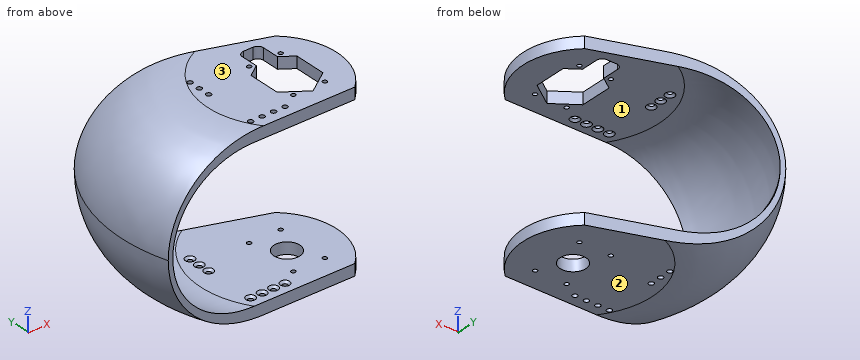
from build123d import *

# Parameters (mm, degrees)
SKETCH1_R                                          = 14.287500000000003
SKETCH1_R_2                                        = 2.3812500000000005
SKETCH1_R_3                                        = 2.3812500000000023
BOSS_EXTRUDE1_DEPTH                                = 190.5
CUT_EXTRUDE1_DEPTH                                 = 314.11990818452256
BOSS_EXTRUDE2_DEPTH                                = 165.1
CUT_EXTRUDE3_REACH                                 = 289.993
FILLET2_R                                          = 82.296
FILLET3_R                                          = 95.25
CSK_FOR_10_FLAT_HEAD_MACHINE_SCREW_100_D           = 5.6134
CSK_FOR_10_FLAT_HEAD_MACHINE_SCREW_100_DEPTH       = 21.30479447
CSK_FOR_10_FLAT_HEAD_MACHINE_SCREW_100_CSINK_D     = 10.16
CSK_FOR_10_FLAT_HEAD_MACHINE_SCREW_100_CSINK_ANGLE = 90


with BuildPart() as part:
    # Sketch1 → Boss-Extrude1 (new body)
    with BuildSketch(Plane.XY):
        with BuildLine():
            Line((31.75000000000027, -53.33999999999999), (-174.9283819167147, -53.33999999999997))
            ThreePointArc((-174.9283819167147, -53.33999999999997), (-179.52896718087996, 34.848878647189125), (-142.26850918824246, 114.91199107732386))
            Line((-142.26850918824246, 114.91199107732386), (31.750000000000263, 54.99261314031172))
            ThreePointArc((31.750000000000263, 54.99261314031172), (55.88000000000002, 0.8263065701558671), (31.75000000000027, -53.33999999999999))
        make_face()
        Circle(SKETCH1_R, mode=Mode.SUBTRACT)
        with Locations((-17.4625, 30.162499999999998)):
            Circle(SKETCH1_R_2, mode=Mode.SUBTRACT)
        with Locations((17.4625, 30.162499999999998)):
            Circle(SKETCH1_R_3, mode=Mode.SUBTRACT)
        with Locations((17.4625, -30.162499999999998)):
            Circle(SKETCH1_R_3, mode=Mode.SUBTRACT)
        with Locations((-17.462499999999995, -30.162499999999998)):
            Circle(SKETCH1_R_2, mode=Mode.SUBTRACT)
    extrude(amount=-BOSS_EXTRUDE1_DEPTH)

    # Sketch2 → Cut-Extrude1 (cut, through all)
    with BuildSketch(Plane.XZ.offset(53.33999999999999)):
        Polygon((-182.87999999999997, -12.7), (55.88000000000002, -12.699999999999989), (55.88000000000004, -177.79999999999998), (-182.87999999999997, -177.79999999999998), align=None)
    extrude(amount=-CUT_EXTRUDE1_DEPTH, mode=Mode.SUBTRACT)


with BuildPart() as cut_extrude1_piece_1:
    # of the separate pieces the step leaves, piece 1, a body of its own (cut_extrude1_pieces)
    add(part.part.solids().sort_by_distance((31.75, 54.99261314, -177.8))[0])



with BuildPart() as cut_extrude1_piece_2:
    # of the separate pieces the step leaves, piece 2, a body of its own (cut_extrude1_pieces)
    add(part.part.solids().sort_by_distance((-142.268509188, 114.911991077, 0))[0])


with BuildPart() as cut_extrude1_piece_1_1:
    add(cut_extrude1_piece_1.part)

    add(cut_extrude1_piece_2.part)  # Boss-Extrude2 merges Cut-Extrude1 piece 2
    # Sketch3 → Boss-Extrude2 (add)
    with BuildSketch(Plane.XY.offset(-177.79999999999998)):
        with BuildLine():
            Line((-142.26850918824255, 114.9119910773238), (-137.46527482419802, 113.25810485268146))
            ThreePointArc((-137.46527482419802, 113.25810485268146), (-174.51803717575487, 34.01402507695267), (-169.84838191671497, -53.33999999999914))
            Line((-169.84838191671497, -53.33999999999914), (-174.92838191671498, -53.339999999999144))
            ThreePointArc((-174.92838191671498, -53.339999999999144), (-179.52896718087993, 34.84887864718949), (-142.26850918824255, 114.9119910773238))
        make_face()
    extrude(amount=BOSS_EXTRUDE2_DEPTH)

    # Sketch5 → Cut-Extrude3 (cut, up to next)
    with BuildSketch(Plane.XY, mode=Mode.PRIVATE) as cut_extrude3_sk1:
        with BuildLine():
            Line((-25.399999999999995, 17.779999999999998), (-25.4, -17.779999999999998))
            Line((-25.4, -17.779999999999998), (9.71e-15, -35.56527147052652))
            Line((9.71e-15, -35.56527147052652), (25.400000000000002, -17.78))
            Line((25.400000000000002, -17.78), (25.400000000000002, 17.779999999999998))
            Line((25.400000000000002, 17.779999999999998), (11.747499999999985, 27.33958341540801))
            Line((11.747499999999985, 27.33958341540801), (11.747499999999983, 46.38958341540796))
            ThreePointArc((11.747499999999983, 46.38958341540796), (9.88762806053456, 50.879711475942585), (5.397499999999937, 52.739583415408006))
            Line((5.397499999999937, 52.739583415408006), (-5.397499999999977, 52.739583415408006))
            ThreePointArc((-5.397499999999977, 52.739583415408006), (-9.887628060534599, 50.879711475942585), (-11.747500000000022, 46.38958341540796))
            Line((-11.747500000000022, 46.38958341540796), (-11.74750000000002, 27.33958341540801))
            Line((-11.74750000000002, 27.33958341540801), (-25.399999999999995, 17.779999999999998))
        make_face()
    cut_extrude3_tool1 = extrude(cut_extrude3_sk1.sketch, amount=-CUT_EXTRUDE3_REACH, mode=Mode.PRIVATE) & cut_extrude1_piece_1_1.part
    add(cut_extrude3_tool1.solids().sort_by_distance((0, 6.295319, 0))[0], mode=Mode.SUBTRACT)

    # Fillet2
    fillet2_edges = [cut_extrude1_piece_1_1.edges().sort_by_distance(p)[0] for p in [
        (-174.51803717575484, 34.014025076952706, -12.699999999999989),
        (-174.51803717575484, 34.014025076952706, -177.79999999999998),
    ]]
    fillet(fillet2_edges, radius=FILLET2_R)

    # Fillet3
    fillet3_edges = [cut_extrude1_piece_1_1.edges().sort_by_distance(p)[0] for p in [
        (-179.52896718087993, 34.848878647189096, -190.5),
        (-179.52896718087993, 34.848878647189096, 0),
    ]]
    fillet(fillet3_edges, radius=FILLET3_R - 0.0001)  # a hair under: the kernel refuses the full size

    # CSK for #10 Flat Head Machine Screw (100)12
    with Locations(Plane(origin=(5.5e-16, 0, -12.69999999999999), x_dir=(-1, 0, 0), z_dir=(0, 0, -1))):
        with Locations((35.228381917, -40.64), (73.328381917, 29.21), (73.328381917, 41.91), (73.328381917, 16.51), (60.628381917, -40.64), (73.328381917, -40.64), (47.928381917, -40.64)):
            csk_for_10_flat_head_machine_screw_100 = CounterSinkHole(CSK_FOR_10_FLAT_HEAD_MACHINE_SCREW_100_D / 2, CSK_FOR_10_FLAT_HEAD_MACHINE_SCREW_100_CSINK_D / 2, depth=CSK_FOR_10_FLAT_HEAD_MACHINE_SCREW_100_DEPTH, counter_sink_angle=CSK_FOR_10_FLAT_HEAD_MACHINE_SCREW_100_CSINK_ANGLE)

    # Mirror1: CSK for #10 Flat Head Machine Screw (100)12 across plane
    add(csk_for_10_flat_head_machine_screw_100.mirror(Plane(origin=(2.08e-15, 0, -95.24999999999999), x_dir=(1, 0, 0), z_dir=(0, 0, -1))), mode=Mode.SUBTRACT)


solid = cut_extrude1_piece_1_1.part
Source: CAD feature listing. Evaluate the final solid. Frame: model axes, mm. Face numbers are marked on the shaded views. Round coordinates to 2 decimals unless told otherwise and drop trailing zeros. Return JSON: item names as keys, results as strings. Group by question number.
1. Section query A-A on y = 41.91. State how many separate pieces and enclosed holes the cut face has, and give its area (3 significant figures).
2. Pin query (flat end, axial travel): pin 1 (1 mm diameter, centred on y = -33.5, z = -109, fed in from -X); pin 2 (1 mm diameter, centred on x = -150, z = -44, fed in from +Y); pin 3 (5 mm diameter, centred on x = -47.93, y = -40.64, fed in from -Z); pin 4 (3 mm diameter, centred on y = 37, z = -103.5, fed in from +X). Return the tip coordinate at first contact, or that it passes through.
3. Material intervals for line 1 along Z through (x, y) = (-55, 33); line 2 along X through (y, z) = (16.5, -9.5); line 3 along Y through (x, z) = (0, -183), sorted ascending. Write a range as from..to.
4. Mould query, pull axis Z, two halves, no side actions, for the marked faces 1, 2 and 3. Classes: released by +Z, released by -Z, zero draft, split by the parting line, or undercut.
Checks:
{
 "1": {"separate pieces": "4", "enclosed holes": "0", "area": "5,000 mm²"},
 "2": {"pin 1": "stops at x = -178.89", "pin 2": "stops at y = 76.68", "pin 3": "passes through", "pin 4": "stops at x = -173.15"},
 "3": {"line 1": "z = -190.5..-177.8, -12.7..0", "line 2": "x = -128.04..-76.14, -70.52..-25.4, 25.4..54.17", "line 3": "y = -53.34..-14.29, 14.29..65.93"},
 "4": {"face 1": "undercut", "face 2": "released by -Z", "face 3": "released by +Z"}
}
